Here's the drawing with two shaded views (mm, measured from the low corner). I have some questions. Coordinates: 2 decimals unless noted, no trailing zeros. Write each loop counter-clockwise with the first axis right and the second up, starting at its lowest first coordinate (ties: lowest second). Pieces come first, ordered by that corner, then holes.
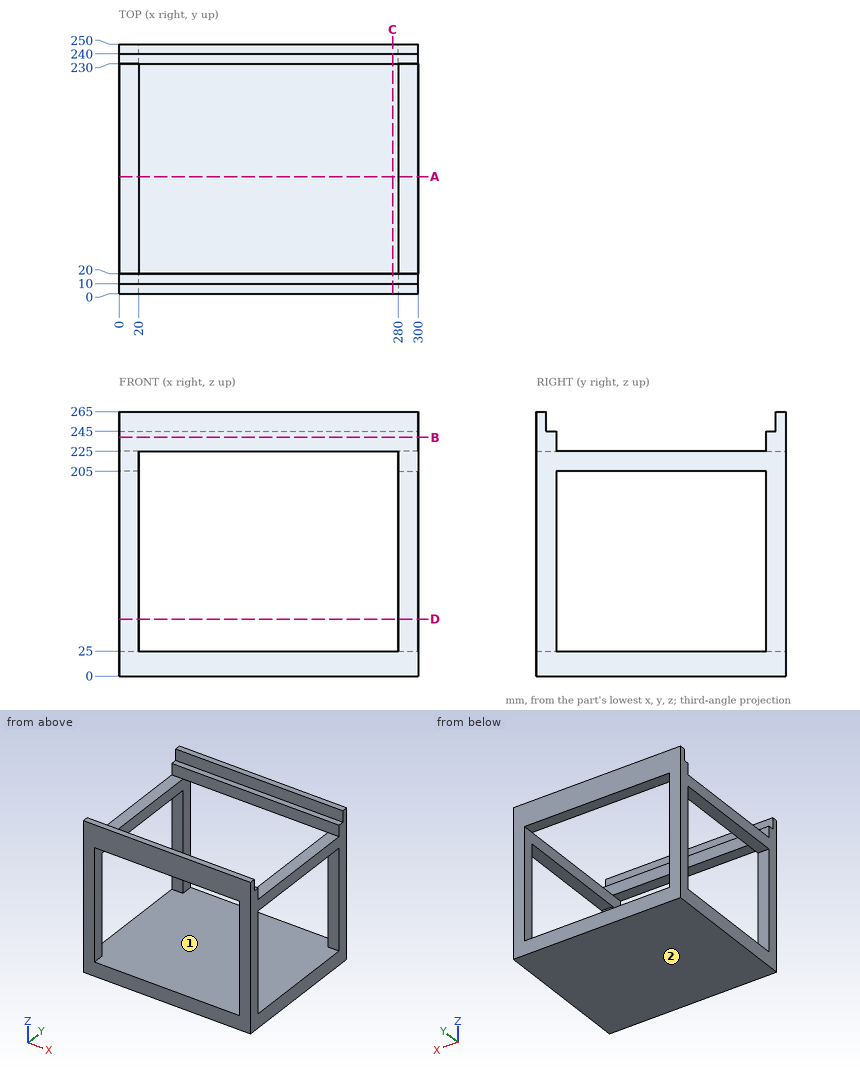
1. If we section it at B-B, the plane z = 239: List the corners of the cut face in (x, y) for me, plus the area to 3 significant figures.
2. I'm going to push flat-ended pins straight in: P1, Ø22, axis at x = 121.5, z = 255.5, coming from the -Y side; P2, Ø5, axis at x = 180.5, y = 233.5, coming from the +Z side; P3, Ø10, axis at x = 11, y = 153.5, coming from the +Z side; P4, Ø3, axis at x = 154.5, y = 48, coming from the +Z side. Where does each tip first touch, or does it pass through?
3. If we section it at D-D, the plane z = 57: List the corners of the cut face in (x, y) for me.
4. We'd pull the mould along X, two halves only. Please class the marked faces 1 and 2: released by +X, released by -X, zero draft, split by the parting line, or undercut.
5. If I drill on L1, parallel to X at y = 150, z = 212.5; L2, parallel to Y at x = 183.5, z = 244; L3, parallel to Z at x = 260, y = 11, over which ranges is the centre line in solid material (lowest first)?
6. If we section it at A-A, the plane y = 117: List the corners of the cut face in (x, z) for me, plus the area to 3 significant figures.
7. If we section it at C-C, the plane x = 274: List the corners of the cut face in (y, z) for me.
Answers:
1. outline: (0, 0) - (300, 0) - (300, 20) - (0, 20) - close; (0, 230) - (300, 230) - (300, 250) - (0, 250) - close
1. area: 12,000 mm2
2. P1: stops at y = 0
2. P2: stops at z = 245
2. P3: stops at z = 225
2. P4: stops at z = 25
3. outline: (0, 0) - (20, 0) - (20, 20) - (0, 20) - close; (0, 230) - (20, 230) - (20, 250) - (0, 250) - close; (280, 0) - (300, 0) - (300, 20) - (280, 20) - close; (280, 230) - (300, 230) - (300, 250) - (280, 250) - close
4. face 1: undercut
4. face 2: zero draft
5. L1: x = 0 to 20, 280 to 300
5. L2: y = 0 to 20, 230 to 250
5. L3: z = 0 to 25, 225 to 245
6. outline: (0, 0) - (300, 0) - (300, 25) - (0, 25) - close; (0, 205) - (20, 205) - (20, 225) - (0, 225) - close; (280, 205) - (300, 205) - (300, 225) - (280, 225) - close
6. area: 8,300 mm2
7. outline: (0, 0) - (250, 0) - (250, 25) - (0, 25) - close; (0, 225) - (20, 225) - (20, 245) - (10, 245) - (10, 265) - (0, 265) - close; (230, 225) - (250, 225) - (250, 265) - (240, 265) - (240, 245) - (230, 245) - close
